from build123d import *

# Parameters (mm, degrees)
SKETCH1_R               = 80
SKETCH1_R_2             = 6
BOSS_EXTRUDE1_DEPTH     = 5
SKETCH3_R               = 80
SKETCH3_R_2             = 65
SKETCH3_R_3             = 13
SKETCH3_R_4             = 6
BOSS_EXTRUDE2_DEPTH     = 13
SKETCH5_R               = 13
SKETCH5_R_2             = 6
BOSS_EXTRUDE3_DEPTH     = 18
CUT_EXTRUDE1_REACH      = 116.56
CUT_EXTRUDE1_END_RADIUS = 13
SKETCH6_R               = 2.5
CHAMFER1_SIZE           = 1
FILLET1_R               = 2


with BuildPart() as part:
    # Sketch1 → Boss-Extrude1 (new, symmetric)
    with BuildSketch(Plane.XY):
        Circle(SKETCH1_R)
        Circle(SKETCH1_R_2, mode=Mode.SUBTRACT)
        with BuildLine():
            Line((14.176102931, 52.905936394), (5.020355656, 18.73622238))
            ThreePointArc((5.020355656, 18.73622238), (4.176125187, 17.575444503), (2.771734362, 17.279105551))
            ThreePointArc((2.771734362, 17.279105551), (0, 17.5), (-2.771734362, 17.279105551))
            ThreePointArc((-2.771734362, 17.279105551), (-4.176125187, 17.575444503), (-5.020355656, 18.73622238))
            Line((-5.020355656, 18.73622238), (-14.176102931, 52.905936394))
            ThreePointArc((-14.176102931, 52.905936394), (-13.558361761, 56.8944703), (-10.196153236, 59.127307221))
            ThreePointArc((-10.196153236, 59.127307221), (0, 60), (10.196153236, 59.127307221))
            ThreePointArc((10.196153236, 59.127307221), (13.558361761, 56.8944703), (14.176102931, 52.905936394))
        make_face(mode=Mode.SUBTRACT)
        with BuildLine():
            Line((19.628620985, 51.134305884), (6.951322155, 18.108813332))
            ThreePointArc((6.951322155, 18.108813332), (6.952030834, 16.673498083), (7.914023213, 15.608274619))
            ThreePointArc((7.914023213, 15.608274619), (10.286241915, 14.157797402), (12.398783618, 12.349905457))
            ThreePointArc((12.398783618, 12.349905457), (13.709143329, 11.76416849), (15.074428242, 12.2070313))
            Line((15.074428242, 12.2070313), (42.566037356, 34.469297408))
            ThreePointArc((42.566037356, 34.469297408), (44.41067566, 38.05918827), (43.003020438, 41.841847871))
            ThreePointArc((43.003020438, 41.841847871), (35.267115138, 48.541019662), (26.505297947, 53.828144876))
            ThreePointArc((26.505297947, 53.828144876), (22.472785499, 53.997998447), (19.628620985, 51.134305884))
        make_face(mode=Mode.SUBTRACT)
        with BuildLine():
            Line((45.935878838, 29.831108518), (16.26783117, 10.564453087))
            ThreePointArc((16.26783117, 10.564453087), (15.424747368, 9.402842107), (15.576892908, 7.975613289))
            ThreePointArc((15.576892908, 7.975613289), (16.643489035, 5.407797402), (17.289918951, 2.703461236))
            ThreePointArc((17.289918951, 2.703461236), (18.005734675, 1.459379963), (19.370581601, 1.015169165))
            Line((19.370581601, 1.015169165), (54.697192278, 2.86655838))
            ThreePointArc((54.697192278, 2.86655838), (58.29962092, 4.686589906), (59.384195451, 8.574224786))
            ThreePointArc((59.384195451, 8.574224786), (57.063390978, 18.541019662), (53.082626196, 27.968460739))
            ThreePointArc((53.082626196, 27.968460739), (49.92009252, 30.476126512), (45.935878838, 29.831108518))
        make_face(mode=Mode.SUBTRACT)
        with BuildLine():
            Line((54.697192278, -2.86655838), (19.370581601, -1.015169165))
            ThreePointArc((19.370581601, -1.015169165), (18.005734675, -1.459379963), (17.289918951, -2.703461236))
            ThreePointArc((17.289918951, -2.703461236), (16.643489035, -5.407797402), (15.576892908, -7.975613289))
            ThreePointArc((15.576892908, -7.975613289), (15.424747368, -9.402842107), (16.26783117, -10.564453087))
            Line((16.26783117, -10.564453087), (45.935878838, -29.831108518))
            ThreePointArc((45.935878838, -29.831108518), (49.92009252, -30.476126512), (53.082626196, -27.968460739))
            ThreePointArc((53.082626196, -27.968460739), (57.063390978, -18.541019662), (59.384195451, -8.574224786))
            ThreePointArc((59.384195451, -8.574224786), (58.29962092, -4.686589906), (54.697192278, -2.86655838))
        make_face(mode=Mode.SUBTRACT)
        with BuildLine():
            Line((42.566037356, -34.469297408), (15.074428242, -12.2070313))
            ThreePointArc((15.074428242, -12.2070313), (13.709143329, -11.76416849), (12.398783618, -12.349905457))
            ThreePointArc((12.398783618, -12.349905457), (10.286241915, -14.157797402), (7.914023213, -15.608274619))
            ThreePointArc((7.914023213, -15.608274619), (6.952030834, -16.673498083), (6.951322155, -18.108813332))
            Line((6.951322155, -18.108813332), (19.628620985, -51.134305884))
            ThreePointArc((19.628620985, -51.134305884), (22.472785499, -53.997998447), (26.505297947, -53.828144876))
            ThreePointArc((26.505297947, -53.828144876), (35.267115138, -48.541019662), (43.003020438, -41.841847871))
            ThreePointArc((43.003020438, -41.841847871), (44.41067566, -38.05918827), (42.566037356, -34.469297408))
        make_face(mode=Mode.SUBTRACT)
        with BuildLine():
            Line((14.176102931, -52.905936394), (5.020355656, -18.73622238))
            ThreePointArc((5.020355656, -18.73622238), (4.176125187, -17.575444503), (2.771734362, -17.279105551))
            ThreePointArc((2.771734362, -17.279105551), (0, -17.5), (-2.771734362, -17.279105551))
            ThreePointArc((-2.771734362, -17.279105551), (-4.176125187, -17.575444503), (-5.020355656, -18.73622238))
            Line((-5.020355656, -18.73622238), (-14.176102931, -52.905936394))
            ThreePointArc((-14.176102931, -52.905936394), (-13.558361761, -56.8944703), (-10.196153236, -59.127307221))
            ThreePointArc((-10.196153236, -59.127307221), (0, -60), (10.196153236, -59.127307221))
            ThreePointArc((10.196153236, -59.127307221), (13.558361761, -56.8944703), (14.176102931, -52.905936394))
        make_face(mode=Mode.SUBTRACT)
        with BuildLine():
            Line((-19.628620985, -51.134305884), (-6.951322155, -18.108813332))
            ThreePointArc((-6.951322155, -18.108813332), (-6.952030834, -16.673498083), (-7.914023213, -15.608274619))
            ThreePointArc((-7.914023213, -15.608274619), (-10.286241915, -14.157797402), (-12.398783618, -12.349905457))
            ThreePointArc((-12.398783618, -12.349905457), (-13.709143329, -11.76416849), (-15.074428242, -12.2070313))
            Line((-15.074428242, -12.2070313), (-42.566037356, -34.469297408))
            ThreePointArc((-42.566037356, -34.469297408), (-44.41067566, -38.05918827), (-43.003020438, -41.841847871))
            ThreePointArc((-43.003020438, -41.841847871), (-35.267115138, -48.541019662), (-26.505297947, -53.828144876))
            ThreePointArc((-26.505297947, -53.828144876), (-22.472785499, -53.997998447), (-19.628620985, -51.134305884))
        make_face(mode=Mode.SUBTRACT)
        with BuildLine():
            Line((-45.935878838, -29.831108518), (-16.26783117, -10.564453087))
            ThreePointArc((-16.26783117, -10.564453087), (-15.424747368, -9.402842107), (-15.576892908, -7.975613289))
            ThreePointArc((-15.576892908, -7.975613289), (-16.643489035, -5.407797402), (-17.289918951, -2.703461236))
            ThreePointArc((-17.289918951, -2.703461236), (-18.005734675, -1.459379963), (-19.370581601, -1.015169165))
            Line((-19.370581601, -1.015169165), (-54.697192278, -2.86655838))
            ThreePointArc((-54.697192278, -2.86655838), (-58.29962092, -4.686589906), (-59.384195451, -8.574224786))
            ThreePointArc((-59.384195451, -8.574224786), (-57.063390978, -18.541019662), (-53.082626196, -27.968460739))
            ThreePointArc((-53.082626196, -27.968460739), (-49.92009252, -30.476126512), (-45.935878838, -29.831108518))
        make_face(mode=Mode.SUBTRACT)
        with BuildLine():
            Line((-54.697192278, 2.86655838), (-19.370581601, 1.015169165))
            ThreePointArc((-19.370581601, 1.015169165), (-18.005734675, 1.459379963), (-17.289918951, 2.703461236))
            ThreePointArc((-17.289918951, 2.703461236), (-16.643489035, 5.407797402), (-15.576892908, 7.975613289))
            ThreePointArc((-15.576892908, 7.975613289), (-15.424747368, 9.402842107), (-16.26783117, 10.564453087))
            Line((-16.26783117, 10.564453087), (-45.935878838, 29.831108518))
            ThreePointArc((-45.935878838, 29.831108518), (-49.92009252, 30.476126512), (-53.082626196, 27.968460739))
            ThreePointArc((-53.082626196, 27.968460739), (-57.063390978, 18.541019662), (-59.384195451, 8.574224786))
            ThreePointArc((-59.384195451, 8.574224786), (-58.29962092, 4.686589906), (-54.697192278, 2.86655838))
        make_face(mode=Mode.SUBTRACT)
        with BuildLine():
            Line((-42.566037356, 34.469297408), (-15.074428242, 12.2070313))
            ThreePointArc((-15.074428242, 12.2070313), (-13.709143329, 11.76416849), (-12.398783618, 12.349905457))
            ThreePointArc((-12.398783618, 12.349905457), (-10.286241915, 14.157797402), (-7.914023213, 15.608274619))
            ThreePointArc((-7.914023213, 15.608274619), (-6.952030834, 16.673498083), (-6.951322155, 18.108813332))
            Line((-6.951322155, 18.108813332), (-19.628620985, 51.134305884))
            ThreePointArc((-19.628620985, 51.134305884), (-22.472785499, 53.997998447), (-26.505297947, 53.828144876))
            ThreePointArc((-26.505297947, 53.828144876), (-35.267115138, 48.541019662), (-43.003020438, 41.841847871))
            ThreePointArc((-43.003020438, 41.841847871), (-44.41067566, 38.05918827), (-42.566037356, 34.469297408))
        make_face(mode=Mode.SUBTRACT)
    extrude(amount=BOSS_EXTRUDE1_DEPTH, both=True)

    # Sketch3 → Boss-Extrude2 (add, symmetric)
    # profile 1 of 2: a face of its own
    with BuildSketch(Plane.XY):
        Circle(SKETCH3_R)
        with Locations(Location((0, 0, 0), (0, 0, 180))):
            Circle(SKETCH3_R_2, mode=Mode.SUBTRACT)
    # profile 2 of 2: a face of its own
    with BuildSketch(Plane.XY):
        with Locations(Location((0, 0, 0), (0, 0, 180))):
            Circle(SKETCH3_R_3)
        Circle(SKETCH3_R_4, mode=Mode.SUBTRACT)
    extrude(amount=BOSS_EXTRUDE2_DEPTH, both=True)

    # Sketch5 → Boss-Extrude3 (add, symmetric)
    with BuildSketch(Plane.XY):
        with Locations(Location((0, 0, 0), (0, 0, 180))):
            Circle(SKETCH5_R)
        Circle(SKETCH5_R_2, mode=Mode.SUBTRACT)
    extrude(amount=BOSS_EXTRUDE3_DEPTH, both=True)

    # Cut-Extrude1: up to this cylinder (the profile starts inside it)
    cut_extrude1_end = Plane(origin=(0, 0, -13), z_dir=(0, 0, -1)) * Cylinder(CUT_EXTRUDE1_END_RADIUS, 260.12, mode=Mode.PRIVATE)
    # Sketch6 → Cut-Extrude1 (cut, up to the surface)
    with BuildSketch(Plane(origin=(0, 0, 0), x_dir=(1, 0, 0), z_dir=(0, 1, 0)), mode=Mode.PRIVATE) as cut_extrude1_sk1:
        with Locations(Location((0, 13, 0), (0, 0, 270))):
            Circle(SKETCH6_R)
    cut_extrude1_tool1 = extrude(cut_extrude1_sk1.sketch, amount=-CUT_EXTRUDE1_REACH, mode=Mode.PRIVATE) & cut_extrude1_end
    add(cut_extrude1_tool1.solids().sort_by_distance((0, 0, -13))[0], mode=Mode.SUBTRACT)

    # Chamfer1
    chamfer1_edges = [part.edges().sort_by_distance(p)[0] for p in [
        (65, 0, 13),
        (65, 0, -13),
    ]]
    chamfer(chamfer1_edges, length=CHAMFER1_SIZE)

    # Fillet1
    fillet1_edges = [part.edges().sort_by_distance(p)[0] for p in [
        (13, 0, -18),
        (13, 0, 18),
    ]]
    fillet(fillet1_edges, radius=FILLET1_R)


solid = part.part
Model file for the job. Use its own axes, mm. A direction names the side the tool comes from. Round coordinates to 2 decimals unless told otherwise and drop trailing zeros.
(1) 3-axis set-ups, long thin cutter, end or side, ignore diameter. For faces 1 (the face through (9.662, 36.06, 0.07)), 2 (the face through (9.3, -9.3, -5)): which of +Z, -Z, +X, -X, +Y, -Y reach the whole face in a straight line?
(2) Pin check, flat tips, straight feed: pin 1 (10 mm diameter, centred on y = -51.5, z = -5, fed in from -X); pin 2 (3 mm diameter, centred on x = -60.5, y = -53, fed in from -Z); pin 3 (1.5 mm diameter, centred on y = -34, z = 11.5, fed in from -X). Stop position of each tip, or through.
(3) Drill centre lines: line 1 (Y direction, x = 0, z = -9); line 2 (Y direction, x = -8, z = -6); line 3 (X direction, y = -38, z = -4.5). Where is each one in solid material? Low to high.
(4) Band-saw the part on A-A (x = 0). Give the number of separate pieces and of enclosed holes in the cut face, then the cut area to 3 significant figures.
Verdict:
1. face 1: +Z, -Z
1. face 2: -Z
2. pin 1: stops at x = -65.1
2. pin 2: stops at z = -13
2. pin 3: stops at x = -72.76
3. line 1: y = -80 to -65, -13 to -6, 6 to 13, 65 to 80
3. line 2: y = -79.6 to -64.51, -10.25 to 10.25, 64.51 to 79.6
3. line 3: x = -70.4 to -44.41, -14.59 to -10.18, 10.18 to 14.59, 44.41 to 70.4
4. separate pieces: 5
4. enclosed holes: 0
4. area: 1,430 mm2
